from build123d import *

# Parameters (mm, degrees)
SKETCH1_W                                         = 164.1
SKETCH1_H                                         = 139
BOSS_EXTRUDE1_DEPTH                               = 3
CSK_FOR_4_FLAT_HEAD_MACHINE_SCREW_100_D           = 3.19999995
CSK_FOR_4_FLAT_HEAD_MACHINE_SCREW_100_CSINK_D     = 5.400000122
CSK_FOR_4_FLAT_HEAD_MACHINE_SCREW_100_CSINK_ANGLE = 90
CUT_EXTRUDE1_REACH                                = 109.571
SKETCH4_R                                         = 2.1
SKETCH4_W                                         = 76.5
SKETCH4_H                                         = 23
CUT_EXTRUDE2_START                                = -3
CUT_EXTRUDE2_DEPTH                                = 3
SKETCH6_W                                         = 164.1
SKETCH6_H                                         = 2
CUT_EXTRUDE3_DEPTH                                = 1.5


with BuildPart() as part:
    # Sketch1 → Boss-Extrude1 (new body)
    with BuildSketch(Plane.XY):
        Rectangle(SKETCH1_W, SKETCH1_H)
    extrude(amount=BOSS_EXTRUDE1_DEPTH)

    # CSK for #4 Flat Head Machine Screw (100)1 (through all)
    with Locations(Plane.XY.offset(3)):
        with Locations((-76.55, 62), (-76.55, 0), (-76.55, -62), (76.55, -62), (76.55, 0), (76.55, 62)):
            CounterSinkHole(CSK_FOR_4_FLAT_HEAD_MACHINE_SCREW_100_D / 2, CSK_FOR_4_FLAT_HEAD_MACHINE_SCREW_100_CSINK_D / 2, counter_sink_angle=CSK_FOR_4_FLAT_HEAD_MACHINE_SCREW_100_CSINK_ANGLE)

    # Sketch4 → Cut-Extrude1 (cut, up to next)
    with BuildSketch(Plane.XY.offset(3), mode=Mode.PRIVATE) as cut_extrude1_sk1:
        with Locations((-15.5, -52)):
            Circle(SKETCH4_R)
    cut_extrude1_tool1 = extrude(cut_extrude1_sk1.sketch, amount=-CUT_EXTRUDE1_REACH, mode=Mode.PRIVATE) & part.part
    # Sketch4 → Cut-Extrude1 (cut, up to next)
    with BuildSketch(Plane.XY.offset(3), mode=Mode.PRIVATE) as cut_extrude1_sk2:
        with Locations((67.1, -52)):
            Circle(SKETCH4_R)
    cut_extrude1_tool2 = extrude(cut_extrude1_sk2.sketch, amount=-CUT_EXTRUDE1_REACH, mode=Mode.PRIVATE) & part.part
    # Sketch4 → Cut-Extrude1 (cut, up to next)
    with BuildSketch(Plane.XY.offset(3), mode=Mode.PRIVATE) as cut_extrude1_sk3:
        with Locations((25.8, -52)):
            Rectangle(SKETCH4_W, SKETCH4_H)
    cut_extrude1_tool3 = extrude(cut_extrude1_sk3.sketch, amount=-CUT_EXTRUDE1_REACH, mode=Mode.PRIVATE) & part.part
    add(cut_extrude1_tool1.solids().sort_by_distance((-15.5, -52, 3))[0], mode=Mode.SUBTRACT)
    add(cut_extrude1_tool2.solids().sort_by_distance((67.1, -52, 3))[0], mode=Mode.SUBTRACT)
    add(cut_extrude1_tool3.solids().sort_by_distance((25.8, -52, 3))[0], mode=Mode.SUBTRACT)

    # Sketch5 → Cut-Extrude2 (cut)
    with BuildSketch(Plane.XY.offset(3).offset(CUT_EXTRUDE2_START)):
        with BuildLine():
            Line((-12.45, -63.5), (-12.45, -40.5))
            ThreePointArc((-12.45, -40.5), (-10.95, -39), (-9.45, -40.5))
            Line((-9.45, -40.5), (-9.45, -63.5))
            ThreePointArc((-9.45, -63.5), (-10.95, -65), (-12.45, -63.5))
        make_face()
        with BuildLine():
            Line((64.05, -63.5), (64.05, -40.5))
            ThreePointArc((64.05, -40.5), (62.55, -39), (61.05, -40.5))
            Line((61.05, -40.5), (61.05, -63.5))
            ThreePointArc((61.05, -63.5), (62.55, -65), (64.05, -63.5))
        make_face()
    extrude(amount=CUT_EXTRUDE2_DEPTH, mode=Mode.SUBTRACT)

    # Sketch6 → Cut-Extrude3 (cut)
    with BuildSketch(Plane(origin=(0, 0, 0), x_dir=(-1, 0, 0), z_dir=(0, 0, -1))):
        with Locations((0, 68.5)):
            Rectangle(SKETCH6_W, SKETCH6_H)
        with Locations((0, -68.5)):
            Rectangle(SKETCH6_W, SKETCH6_H)
    extrude(amount=-CUT_EXTRUDE3_DEPTH, mode=Mode.SUBTRACT)


solid = part.part
Design review of the part built by this model. Coordinates are the model's own, in mm. Give positions to 0.01 mm unless a question says otherwise; leave off trailing zeros. Write each loop counter-clockwise with the first axis right and the second up, starting at its lowest first coordinate (ties: lowest second). Pieces come first, ordered by that corner, then holes. Notation, with made-up numbers: M 38.25,37.25 L 46.25,37.25 A16 ccw 46.25,47.25 Z; hole C 85,19 d11. An arc over 180 degrees is marked long. Return JSON: item names as keys, results as strings. Group by question number.
Item 1: Take a section at B-B (y = -56). Give the boundary of the cut face in (x, z).
Item 2: Take a section at C-C (x = 46). Give the boundary of the cut face in (y, z).
Item 3: Wall thickness on line 1 along X through (y, z) = (0, 1.55); line 2 along Y through (x, z) = (76.55, 1.45); line 3 along X through (y, z) = (-62, 1.05): over which ranges is each line inside the solid? List them lowest first.
Item 4: The part is to be moulded in two halves that separate along X. For faces 1 (the flat face through (-1, 1, 0)), 2 (the cylindrical face through (-15.96, -54.05, 1.52)), say which applies: pulls with the +X half, pulls with the -X half, needs draft (parallel to the pull), parting line crosses it, or undercut.
Item 5: Take a section at A-A (x = 67.1). Give the boundary of the cut face in (y, z), plus the area to 3 significant figures.
Item 6: Clearance check with flat-ended pins moving along their axes: pin 1 Ø1.6 at (x, y) = (-31.5, 68.5) entering from -Z; pin 2 Ø3.5 at (x, y) = (76.55, 0) entering from +Z. State where each tip first meets the part, or that it passes through.
Return value:
{
 "1": {"outline": "M -82.05,0 L -12.45,0 L -12.45,3 L -82.05,3 Z; M 64.05,0 L 82.05,0 L 82.05,3 L 64.05,3 Z"},
 "2": {"outline": "M -69.5,1.5 L -67.5,1.5 L -67.5,0 L -63.5,0 L -63.5,3 L -69.5,3 Z; M -40.5,0 L 67.5,0 L 67.5,1.5 L 69.5,1.5 L 69.5,3 L -40.5,3 Z"},
 "3": {"line 1": "x = -82.05 to -78.15, -74.95 to 74.95, 78.15 to 82.05", "line 2": "y = -67.5 to -63.6, -60.4 to -1.6, 1.6 to 60.4, 63.6 to 67.5", "line 3": "x = -82.05 to -78.15, -74.95 to -12.45, 64.05 to 74.95, 78.15 to 82.05"},
 "4": {"face 1": "needs draft", "face 2": "undercut"},
 "5": {"outline": "M -69.5,1.5 L -67.5,1.5 L -67.5,0 L -54.1,0 L -54.1,3 L -69.5,3 Z; M -49.9,0 L 67.5,0 L 67.5,1.5 L 69.5,1.5 L 69.5,3 L -49.9,3 Z", "area": "398 mm2"},
 "6": {"pin 1": "stops at z = 1.5", "pin 2": "stops at z = 2.05"}
}
